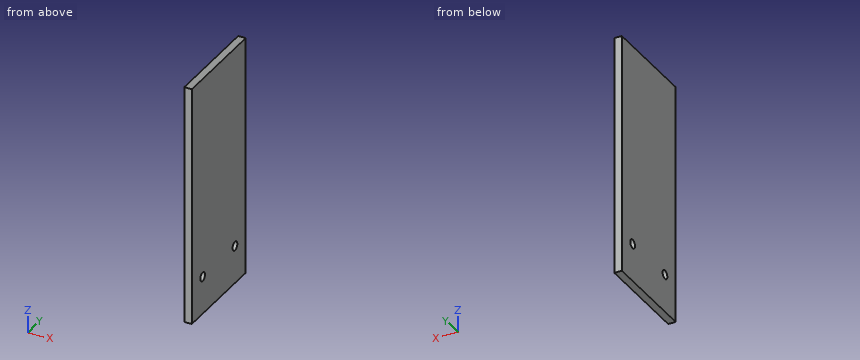
Autodesk Inventor part; units mm, degrees
ref_plane "Start Plane" through (0, 0, 0) normal (0, 0, 1) x (1, 0, 0)
ref_plane "End Plane" through (0, 0, 475) normal (0, 0, 1) x (1, 0, 0)
ref_plane "YZ Plane" through (0, 0, 0) normal (1, 0, 0) x (0, 1, 0)
ref_plane "Start Plane" through (0, 0, 0) normal (0, 0, 1) x (1, 0, 0)
ref_plane "End Plane" through (0, 0, 475) normal (0, 0, 1) x (1, 0, 0)
sketch "Sketch" plane through (0, 0, 0) normal (0, 0, 1) x (1, 0, 0)
  line L0 (7.5, -100) -> (-7.5, -100)
  line L1 (-7.5, -100) -> (-7.5, 100)
  line L2 (-7.5, 100) -> (7.5, 100)
  line L3 (7.5, 100) -> (7.5, -100)
  line L4 (-6, 0) -> (8, 0) construction
  line L5 (0, -30) -> (0, 40) construction
  line L6 (0, 140) -> (0, -140) construction
  line L7 (-11, 0) -> (13.5, 0) construction
  dimension "d0" = 200
  dimension "d1" = 15
  dimension "d4" = 7.5
  dimension "d5" = 100
extrude "Body" add sketch "Sketch" along normal up to surface (475 mm away) from surface at 0
sketch "Sketch3" plane through (0, 0, 0) normal (0, 0, 1) x (1, 0, 0)
  line L0 (0, 0) -> (10, 0)
ref_plane "Work Plane3" through (0, 0, 0) normal (0, -1, 0) x (1, 0, 0)
sketch "Sketch5" plane through (-7.5, 100, 0) normal (-1, 0, 0) x (0, 0, 1)
  point P0 (75, -40)
hole "Hole1" at (-7.5, 60, 75) direction (1, 0, 0) diameter 17.5 end through all
sketch "Sketch6" plane through (-7.5, 100, 0) normal (-1, 0, 0) x (0, 0, 1)
  point P0 (75, -160)
hole "Hole2" at (-7.5, -60, 75) direction (1, 0, 0) diameter 17.5 end through all
sketch "Sketch4" plane through (0, 0, 0) normal (0, -1, 0) x (1, 0, 0)
  line L0 (-2, 0) -> (12, 0)
  line L1 (-2, 475) -> (12, 475)
  dimension "d9" = 475
equation "\"d0\" = G_W"
equation "\"d1\" = G_H"
equation "\"d4\" = 0.5 * d1"
equation "\"d5\" = 0.5 * d0"
equation "\"d2\" = G_L"
equation "\"G_W\" = 200"
equation "\"G_H\" = 15"
equation "\"G_L\" = d9"
equation "\"G_OFFSET_START\" = 0"
equation "\"G_OFFSET_END\" = 0"
equation "\"d7\" = G_OFFSET_END + B_L"
equation "\"B_L\" = 475"
properties part number "DIN EN 10278 - 200 x 15 - 475" material "Steel, Mild"
CAD build for the part. Positions are in the model's coordinates, mm. Round coordinates to 2 decimals unless told otherwise and drop trailing zeros. Loops run counter-clockwise (first coordinate to the right, second up) from the corner with the lowest first, then second, coordinate; pieces in that order, holes last. Notation, with made-up numbers: (-18, 80.25) - (23, 80.25) arc R25 cw to (23, 107.25) - close; hole circle Ø5 at (63, -10.5). An arc over 180 degrees is marked (long way). Return JSON: item names as keys, results as strings. Group by question number.
Q1. Drill centre lines: line 1 along Y through (x, z) = (2, 75); line 2 along Z through (x, y) = (2, 60); line 3 along Z through (x, y) = (2.5, 56.5). Where is each one in solid material? Low to high. Write a range as [from, to].
Q2. Band-saw the part on B-B on z = 75. Give the cut face in (x, y).
Q3. Flat gauge pins, fed straight in: pin 1 Ø16 at (y, z) = (60, 75) entering from +X; pin 2 Ø20 at (y, z) = (-60, 75) entering from +X. Where does each tip first touch, or does it go through?
Q4. Band-saw the part on A-A on y = -60. Give the cut face in (x, z), plus the area to 3 significant figures.
Solutions:
{
 "1": {"line 1": "y = [-100, -68.75], [-51.25, 51.25], [68.75, 100]", "line 2": "z = [0, 66.25], [83.75, 475]", "line 3": "z = [0, 66.98], [83.02, 475]"},
 "2": {"outline": "(-7.5, -100) - (7.5, -100) - (7.5, -68.75) - (-7.5, -68.75) - close; (-7.5, -51.25) - (7.5, -51.25) - (7.5, 51.25) - (-7.5, 51.25) - close; (-7.5, 68.75) - (7.5, 68.75) - (7.5, 100) - (-7.5, 100) - close"},
 "3": {"pin 1": "passes through", "pin 2": "stops at x = 7.5"},
 "4": {"outline": "(-7.5, 0) - (7.5, 0) - (7.5, 66.25) - (-7.5, 66.25) - close; (-7.5, 83.75) - (7.5, 83.75) - (7.5, 475) - (-7.5, 475) - close", "area": "6,860 mm^2"}
}
